from build123d import *

# Parameters (mm, degrees)
BOSS_EXTRUDE1_DEPTH      = 88.9
BOSS_EXTRUDE2_DEPTH      = 31.75
BOSS_EXTRUDE2_DEPTH_BACK = 31.75


with BuildPart() as part:
    # Sketch2 → Boss-Extrude1 (new body)
    with BuildSketch(Plane.XY):
        with BuildLine():
            Line((90.17, 0), (67.31, 0))
            ThreePointArc((67.31, 0), (72.367383476, 4.152406467), (78.74, 5.6388))
            ThreePointArc((78.74, 5.6388), (85.112616524, 4.152406467), (90.17, 0))
        make_face()
    extrude(amount=-BOSS_EXTRUDE1_DEPTH)

    # Sketch3 → Boss-Extrude2 (add, two sides)
    with BuildSketch(Plane.XY.offset(-44.45)) as boss_extrude2_sk:
        with BuildLine():
            Line((40.64, 65.991135768), (75.674904681, 5.308900822))
            ThreePointArc((75.674904681, 5.308900822), (73.244625787, 4.48173949), (70.942491559, 3.345680792))
            Line((70.942491559, 3.345680792), (40.64, 55.831135768))
            Line((40.64, 55.831135768), (40.64, 65.991135768))
        make_face()
    extrude(amount=BOSS_EXTRUDE2_DEPTH)
    extrude(boss_extrude2_sk.sketch, amount=-BOSS_EXTRUDE2_DEPTH_BACK)


solid = part.part
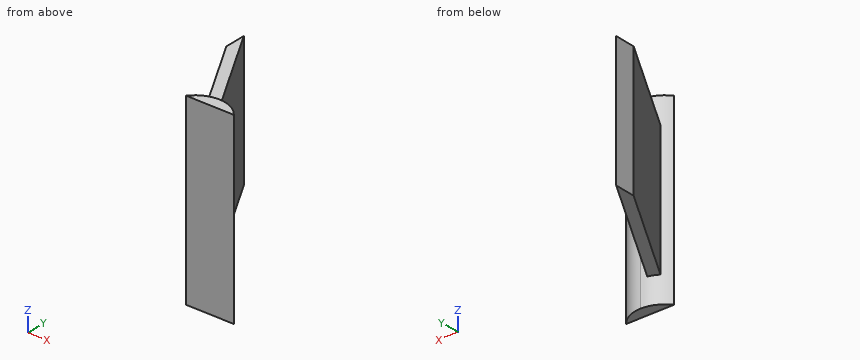
Verification items for the finished model (mm, model axes). Coordinates: 2 decimals unless noted, no trailing zeros. Order: outer loops, then holes, each group sorted by start corner. A loop starts at its lowest first (then second) coordinate and runs counter-clockwise, first axis right, second up. Notation, with made-up numbers: M 61.5,38.25 L 88.5,38.25 A20 ccw 88.5,61.25 Z; hole C -20.75,-13 d8. An arc over 180 degrees is marked long. One line per item, written item: value. Start each with the question number.
Item 1: Sectioned sample at A-A on x = 68.5. Record the cut outline in (y, z), then the cut area to 3 significant figures.
Item 2: Thickness scan on probe 1 along X at (y, z) = (9.5, -22); probe 2 along X at (y, z) = (9, -66); probe 3 along Y at (x, z) = (46, -69). Record the ranges inside material, lowest first.
Item 3: Sectioned sample at D-D on z = -7.5. Record the cut outline in (x, y), then the cut area to 3 significant figures.
Item 4: Depth check by flat-ended pin: P1, Ø17.5, axis at x = 57, y = 30.5, coming from the -Z side; P2, Ø3, axis at x = 46.5, z = -28.5, coming from the +Y side; P3, Ø1.5, axis at x = 46.5, y = 52.5, coming from the +Z side. Enter the tip coordinate at first touch or a pass-through.
Item 5: Sectioned sample at B-B on z = -34.5. Record the cut outline in (x, y).
Item 6: Sectioned sample at C-C on y = 7. Record the cut outline in (x, z).
Calculated:
1. outline: M 0,-88.9 L 1.36,-88.9 L 1.36,0 L 0,0 Z; M 7.58,-76.2 L 17.74,-76.2 L 17.74,-12.7 L 7.58,-12.7 Z
1. area: 766 mm^2
2. probe 1: 67.39 to 73.26
2. probe 2: 67.68 to 73.54
2. probe 3: 46.55 to 56.71
3. outline: M 67.31,0 L 90.17,0 A14.4 ccw Z
3. area: 90.0 mm^2
4. P1: z = -76.2
4. P2: y = 58.44
4. P3: z = -12.7
5. outline: M 40.64,55.83 L 70.94,3.35 A14.4 ccw 67.31,0 L 90.17,0 A14.4 ccw 75.67,5.31 L 40.64,65.99 Z
6. outline: M 68.83,-76.2 L 74.7,-76.2 L 74.7,-12.7 L 68.83,-12.7 Z
